Geometry: final body of the model. Coordinates: model frame, mm. Face numbers are marked on the shaded views. A direction names the side the tool comes from. Coordinates: 2 decimals unless noted, no trailing zeros. Loops run counter-clockwise (first coordinate to the right, second up) from the corner with the lowest first, then second, coordinate; pieces in that order, holes last. Notation, with made-up numbers: (-6.75, 58.5) - (41.25, 58.5) arc R26 cw to (41.25, 90.5) - close; hole circle Ø11 at (1, -24). An arc over 180 degrees is marked (long way). Answer in a Markdown table with one row per item.
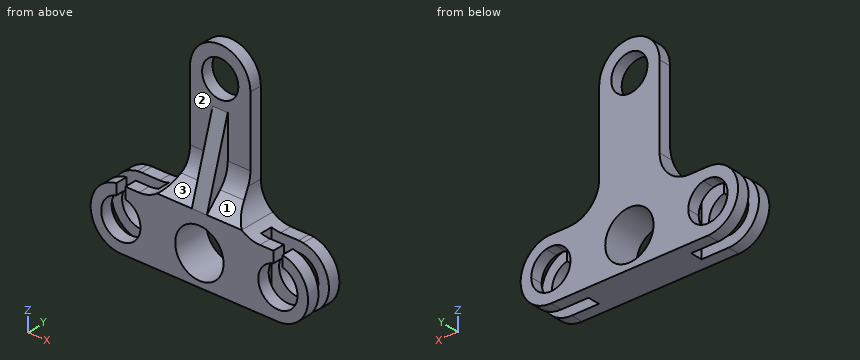
from build123d import *

# Parameters (mm, degrees)
F0_R     = 4
F0_R_2   = 3
F1_DEPTH = 6
F3_DEPTH = 12.5
F5_DEPTH = 1.25
F6_W     = 9.5
F6_H     = 2
F7_DEPTH = 25
F9_DEPTH = 3


with BuildPart() as f1:
    # F0 (on Front) → F1 (new body)
    with BuildSketch(Plane.XZ):
        with BuildLine():
            ThreePointArc((-12.25, 3.162278), (-10.45049, 2.015564), (-9.75, 0))
            ThreePointArc((-9.75, 0), (-15.015564, -2.54951), (-13.75, 3.162278))
            Line((-13.75, 3.162278), (-13.75, 4.94343))
            ThreePointArc((-13.75, 4.94343), (-17.985837, -0.376065), (-13, -5))
            Line((-13, -5), (13, -5))
            ThreePointArc((13, -5), (17.985837, -0.376065), (13.75, 4.94343))
            Line((13.75, 4.94343), (13.75, 3.162278))
            ThreePointArc((13.75, 3.162278), (15.54951, 2.015564), (16.25, 0))
            ThreePointArc((16.25, 0), (10.984436, -2.54951), (12.25, 3.162278))
            Line((12.25, 3.162278), (12.25, 5))
            Line((12.25, 5), (10, 5))
            ThreePointArc((10, 5), (8.418861, 5.256584), (7, 6))
            Line((7, 6), (1.25, 6))
            Line((1.25, 6), (-1.25, 6))
            Line((-1.25, 6), (-7, 6))
            ThreePointArc((-7, 6), (-8.418861, 5.256584), (-10, 5))
            Line((-10, 5), (-12.25, 5))
            Line((-12.25, 5), (-12.25, 3.162278))
        make_face()
        Circle(F0_R, mode=Mode.SUBTRACT)
        with BuildLine():
            ThreePointArc((-13.75, 3.162278), (-13, 3.25), (-12.25, 3.162278))
            Line((-12.25, 3.162278), (-12.25, 5))
            Line((-12.25, 5), (-13, 5))
            ThreePointArc((-13, 5), (-13.376065, 4.985837), (-13.75, 4.94343))
            Line((-13.75, 4.94343), (-13.75, 3.162278))
        make_face()
        with BuildLine():
            ThreePointArc((-5, 10), (-5.527864, 7.763932), (-7, 6))
            Line((-7, 6), (-1.25, 6))
            Line((-1.25, 6), (-1.25, 19))
            Line((-1.25, 19), (1.25, 19))
            Line((1.25, 19), (1.25, 6))
            Line((1.25, 6), (7, 6))
            ThreePointArc((7, 6), (5.527864, 7.763932), (5, 10))
            Line((5, 10), (5, 23.5))
            ThreePointArc((5, 23.5), (0, 28.5), (-5, 23.5))
            Line((-5, 23.5), (-5, 10))
        make_face()
        with Locations((0, 23.5)):
            Circle(F0_R_2, mode=Mode.SUBTRACT)
        with BuildLine():
            Line((13.75, 3.162278), (13.75, 4.94343))
            ThreePointArc((13.75, 4.94343), (13.376065, 4.985837), (13, 5))
            Line((13, 5), (12.25, 5))
            Line((12.25, 5), (12.25, 3.162278))
            ThreePointArc((12.25, 3.162278), (13, 3.25), (13.75, 3.162278))
        make_face()
    extrude(amount=F1_DEPTH)

    # F2 (on Right) → F3 (cut, symmetric)
    with BuildSketch(Plane.YZ):
        Polygon((-2, 19.08341), (-2, 28.5), (-6, 28.5), (-6, 6), align=None)
        with BuildLine():
            Line((-2, 12.071068), (-2, 19.08341))
            Line((-2, 19.08341), (-6, 6))
            Line((-6, 6), (-3.464466, 8.535534))
            ThreePointArc((-3.464466, 8.535534), (-2.380602, 10.157651), (-2, 12.071068))
        make_face()
    extrude(amount=F3_DEPTH, both=True, mode=Mode.SUBTRACT)

    # F4 (on Right) → F5 (join, symmetric)
    with BuildSketch(Plane.YZ):
        Polygon((-2, 19.08341), (-6, 6), (0, 6), (0, 19.08341), align=None)
    extrude(amount=F5_DEPTH, both=True)

    # F6 (on face) → F7 (cut)
    with BuildSketch(Plane(origin=(0, 0, -5), x_dir=(1, 0, 0), z_dir=(0, 0, -1))):
        with Locations((-13.25, 3)):
            Rectangle(F6_W, F6_H)
        with Locations((13.25, 3)):
            Rectangle(F6_W, F6_H)
    extrude(amount=-F7_DEPTH, mode=Mode.SUBTRACT)

    # F8 (on face) → F9 (cut)
    with BuildSketch(Plane.XZ.offset(6)):
        with BuildLine():
            Line((-12.25, 3.162278), (-12.25, 5))
            Line((-12.25, 5), (-13, 5))
            ThreePointArc((-13, 5), (-13.376065, 4.985837), (-13.75, 4.94343))
            Line((-13.75, 4.94343), (-13.75, 3.162278))
            ThreePointArc((-13.75, 3.162278), (-13, 3.25), (-12.25, 3.162278))
        make_face()
        with BuildLine():
            Line((13, 5), (12.25, 5))
            Line((12.25, 5), (12.25, 3.162278))
            ThreePointArc((12.25, 3.162278), (13, 3.25), (13.75, 3.162278))
            Line((13.75, 3.162278), (13.75, 4.94343))
            ThreePointArc((13.75, 4.94343), (13.376065, 4.985837), (13, 5))
        make_face()
    extrude(amount=-F9_DEPTH, mode=Mode.SUBTRACT)


solid = f1.part
(1) Access query for the marked faces 1, 2 and 3. Directions: +Z, -Z, +X, -X, +Y, -Y. A direction counts if a zero-diameter tool reaches every point of the face in a straight line with its end or side. Return the directions, or none.
Verdict:
| item | result |
|---|---|
| face 1 | +Z, +X, -Y |
| face 2 | +Z, -Y |
| face 3 | +Z, -X, -Y |
(2) Cut plane C-C on y = -1. Output: boundary loops of the cut face in (x, z).
Verdict:
| item | result |
|---|---|
| outline | (-13.75, 4.94) arc R5 ccw to (-13, -5) - (13, -5) arc R5 ccw to (13.75, 4.94) arc R5 ccw to (13, 5) - (10, 5) arc R5 cw to (7, 6) arc R5 cw to (5, 10) - (5, 23.5) arc R5 ccw to (-5, 23.5) - (-5, 10) arc R5 cw to (-7, 6) arc R5 cw to (-10, 5) - (-13, 5) arc R5 ccw to start; hole (-13.75, 3.16) arc R3.25 ccw (long way) to (-12.25, 3.16) arc R3.25 ccw to start; hole circle Ø8 at (0, 0); hole circle Ø6 at (0, 23.5); hole (12.25, 3.16) arc R3.25 ccw (long way) to (13.75, 3.16) arc R3.25 ccw to start |
(3) First-contact query: pin 1 Ø0.6 at (y, z) = (-5, 4.5) entering from +X; pin 2 Ø4 at (x, z) = (13, 0) entering from -Y; pin 3 Ø2 at (x, y) = (12, -1) entering from +Z; pin 4 Ø1.5 at (y, z) = (-3.5, 12) entering from -X. Flat tips, straight axial feed; report the tip coordinate or a pass-through.
Verdict:
| item | result |
|---|---|
| pin 1 | stops at x = 15.71 |
| pin 2 | passes through |
| pin 3 | stops at z = 5 |
| pin 4 | stops at x = -1.25 |
(4) Cut plane D-D on z = 23. Output: boundary loops of the cut face in (x, y), then the cut area to 3 significant figures.
Verdict:
| item | result |
|---|---|
| outline | (-5, -2) - (-2.96, -2) - (-2.96, 0) - (-5, 0) - close; (2.96, -2) - (5, -2) - (5, 0) - (2.96, 0) - close |
| area | 8.17 mm² |
(5) Cut plane A-A on z = -1. State how many separate pieces and enclosed holes the cut face has, then the cut area to 3 significant figures.
Verdict:
| item | result |
|---|---|
| separate pieces | 6 |
| enclosed holes | 0 |
| area | 81.2 mm² |
(6) Ray query, probe 1 along Z at (x, y) = (13, -1.1); probe 2 along Y at (x, z) = (-11, -4); probe 3 along X at (y, z) = (-5, 0.5). Return the intervals inside material, ascending.
Verdict:
| item | result |
|---|---|
| probe 1 | z = -5 to -3.25, 3.25 to 5 |
| probe 2 | y = -6 to -4, -2 to 0 |
| probe 3 | x = -17.97 to -16.21, -9.79 to -3.97, 3.97 to 9.79, 16.21 to 17.97 |
(7) Cut plane B-B on x = 0. Output: boundary loops of the cut face in (y, z), then the cut area to 3 significant figures.
Verdict:
| item | result |
|---|---|
| outline | (-6, -5) - (0, -5) - (0, -4) - (-6, -4) - close; (-6, 4) - (0, 4) - (0, 20.5) - (-2, 20.5) - (-2, 19.08) - (-6, 6) - close; (-2, 26.5) - (0, 26.5) - (0, 28.5) - (-2, 28.5) - close |
| area | 77.2 mm² |
